Can you work these out from the model? Positions are in its coordinate system, mm. Give positions to 0.01 mm unless a question says otherwise; leave off trailing zeros. Loops run counter-clockwise (first coordinate to the right, second up) from the corner with the lowest first, then second, coordinate; pieces in that order, holes last. Notation, with made-up numbers: (31.5, 37.25) - (41.5, 37.25) arc R23 ccw to (41.5, 48.25) - close; hole circle Ø7 at (26.5, 74). An arc over 180 degrees is marked (long way). Answer as a JSON object with one key per item and string values. Group by question number.
Item 1: Suppose I cut it at A-A on y = 3.25. Write out the boundary of the cut face in (x, z).
Item 2: Will these pins go through, and if not, where does the flat tip stop? pin 1 (10 mm diameter, centred on x = -16, z = -30.5, fed in from +Y); pin 2 (4 mm diameter, centred on y = 5, z = -35, fed in from -X); pin 3 (0.5 mm diameter, centred on y = 1, z = -6.5, fed in from +X).
Item 3: Suppose I cut it at D-D on x = -17.75. Write out the boundary of the cut face in (y, z).
Item 4: Suppose I cut it at B-B on z = -42. Write out the boundary of the cut face in (x, y) (1 decimal), and give its area (3 significant figures).
Item 5: Suppose I cut it at C-C on y = 1.25. Write out the boundary of the cut face in (x, z), and give its area (3 significant figures).
Item 6: Please list where these lines run through material, in increasing order: L1, parallel to Z at x = 0.5, y = 5.5; L2, parallel to Y at x = -16.5, z = -8; L3, parallel to X at y = 4.5, z = -30.
from build123d import *

# Parameters (mm, degrees)
EXTRUDE1_DEPTH     = 50.8
SKETCH2_W          = 6.8326
SKETCH2_H          = 25.4
CUT_EXTRUDE4_DEPTH = 56.557383842


with BuildPart() as part:
    # Sketch1 → Extrude1 (new body)
    with BuildSketch(Plane.XY):
        with BuildLine():
            Line((-21.43125, 0), (0, 0))
            ThreePointArc((0, 0), (1.779677423, 6.332436821), (-3.038247732, 1.8542))
            Line((-3.038247732, 1.8542), (-1.378132955, 2.628324234))
            ThreePointArc((-1.378132955, 2.628324234), (0.796631885, 4.789447439), (0, 1.8288))
            Line((0, 1.8288), (-21.43125, 1.8288))
            Line((-21.43125, 1.8288), (-21.43125, 0))
        make_face()
    extrude(amount=-EXTRUDE1_DEPTH)

    # Sketch2 → Cut-Extrude4 (cut, through all)
    with BuildSketch(Plane(origin=(0, 0, 0), x_dir=(1, 0, 0), z_dir=(0, 1, 0))):
        with Locations((0, 12.7)):
            Rectangle(SKETCH2_W, SKETCH2_H)
    extrude(amount=CUT_EXTRUDE4_DEPTH, mode=Mode.SUBTRACT)


solid = part.part
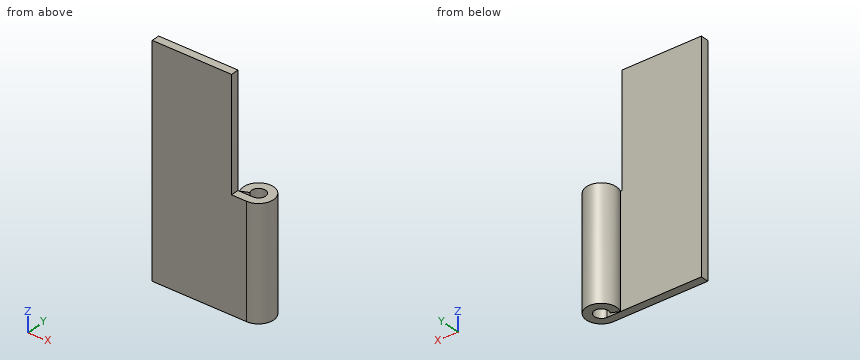
Worked out:
{
 "1": {"outline": "(-3.41, -50.8) - (-1.58, -50.8) - (-1.58, -25.4) - (-3.41, -25.4) - close; (1.58, -50.8) - (3.41, -50.8) - (3.41, -25.4) - (1.58, -25.4) - close"},
 "2": {"pin 1": "stops at y = 1.83", "pin 2": "stops at x = -3.42", "pin 3": "stops at x = -3.42"},
 "3": {"outline": "(0, -50.8) - (1.83, -50.8) - (1.83, 0) - (0, 0) - close"},
 "4": {"outline": "(-21.4, 0) - (0, 0) arc R3.4 ccw (long way) to (-3, 1.9) - (-1.4, 2.6) arc R1.6 cw (long way) to (0, 1.8) - (-21.4, 1.8) - close", "area": "63.0 mm2"},
 "5": {"outline": "(-21.43, -50.8) - (2.64, -50.8) - (2.64, -25.4) - (-3.42, -25.4) - (-3.42, 0) - (-21.43, 0) - close", "area": "1,070 mm2"},
 "6": {"L1": "z = -50.8 to -25.4", "L2": "y = 0 to 1.83", "L3": "x = -3.24 to -1.16, 1.16 to 3.24"}
}
